Check sheet for the modelled part. Datum: model origin and axes. Units: mm. A direction names the side the tool comes from. Round coordinates to 2 decimals unless told otherwise and drop trailing zeros. Order: outer loops, then holes, each group sorted by start corner. A loop starts at its lowest first (then second) coordinate and runs counter-clockwise, first axis right, second up.
Q1. Mould release check, pull along Z, two halves, no side actions. Record for faces 1 (the cylindrical face through (-15.2, -5.73, 58.03)), 2 (the flat face through (14.3, 0, 27)): +Z half, -Z half, draft (parallel to the pull), parting line (faces both ways), or undercut.
Q2. Set-up check for faces 3 (the flat face through (-15.8, 0, -3)), 4 (the flat face through (0, 6.3, -3)), 5 (the cylindrical face through (-13.73, 4.7, 27.88)), 6 (the flat face through (0, 3.8, 28)): record each of +Z, -Z, +X, -X, +Y, -Y from which the full face is reachable in a straight line by a thin tool's end or side.
Q3. Cross-section at A-A on x = -6.5. Record the cut outline in (y, z), then the cut area to 3 significant figures.
Q4. Cross-section at D-D on y = 8. Record the cut outline in (x, z).
Q5. Cross-section at B-B on z = 35. Record the cut outline in (x, y).
Q6. Scan lines: probe 1 along X at (y, z) = (2, 53.5); probe 2 along Y at (x, z) = (-3, 37.5); probe 3 along Z at (x, y) = (-9, 5.75). Record each from-to range of solid material in increasing order.
Q7. Cross-section at C-C on y = -1. Record the cut outline in (x, z).
Q8. Depth check by flat-ended pin: P1, Ø8, axis at y = -0.5, z = 36.5, coming from the -X side; P2, Ø2, axis at x = 4, z = 58.5, coming from the -Y side; P3, Ø3, axis at y = 1, z = -3.5, coming from the +X side; P4, Ø6, axis at x = -1, y = 0, coming from the +Z side. Enter the tip coordinate at first touch or a pass-through.
from build123d import *

# Parameters (mm, degrees)
SKETCH1_W           = 28.6
SKETCH1_H           = 10.6
SKETCH1_W_2         = 25.6
SKETCH1_H_2         = 7.6
BOSS_EXTRUDE1_DEPTH = 55
SKETCH2_W           = 36.6
SKETCH2_H           = 18.6
SKETCH2_W_2         = 25.6
SKETCH2_H_2         = 7.6
BOSS_EXTRUDE3_DEPTH = 1
SKETCH3_W           = 31.6
SKETCH3_H           = 12.6
SKETCH3_W_2         = 25.6
SKETCH3_H_2         = 7.6
BOSS_EXTRUDE4_DEPTH = 4
FILLET1_R           = 2
FILLET2_R           = 2


with BuildPart() as part:
    # Sketch1 → Boss-Extrude1 (new body)
    with BuildSketch(Plane.XY):
        Rectangle(SKETCH1_W, SKETCH1_H)
        Rectangle(SKETCH1_W_2, SKETCH1_H_2, mode=Mode.SUBTRACT)
    extrude(amount=BOSS_EXTRUDE1_DEPTH)

    # Sketch2 → Boss-Extrude3 (add)
    with BuildSketch(Plane.XY.offset(55)):
        Rectangle(SKETCH2_W, SKETCH2_H)
        Rectangle(SKETCH2_W_2, SKETCH2_H_2, mode=Mode.SUBTRACT)
    boss_extrude3 = extrude(amount=BOSS_EXTRUDE3_DEPTH)

    # Sketch3 → Boss-Extrude4 (add)
    with BuildSketch(Plane.XY.offset(56)):
        Rectangle(SKETCH3_W, SKETCH3_H)
        Rectangle(SKETCH3_W_2, SKETCH3_H_2, mode=Mode.SUBTRACT)
    boss_extrude4 = extrude(amount=BOSS_EXTRUDE4_DEPTH)

    # Mirror1: Boss-Extrude3, Boss-Extrude4 across plane
    add(boss_extrude3.mirror(Plane(origin=(0, 0, 27.5), x_dir=(1, 0, 0), z_dir=(0, 0, -1))))
    add(boss_extrude4.mirror(Plane(origin=(0, 0, 27.5), x_dir=(1, 0, 0), z_dir=(0, 0, -1))))

    # Fillet1
    fillet1_edges = [part.edges().sort_by_distance(p)[0] for p in [
        (12.8, -3.8, 27.5),
        (12.8, 3.8, 27.5),
        (-12.8, 3.8, 27.5),
        (-12.8, -3.8, 27.5),
        (15.8, -6.3, 58),
        (15.8, 6.3, 58),
        (-15.8, 6.3, 58),
        (-15.8, -6.3, 58),
        (14.3, -5.3, 27.5),
        (-14.3, -5.3, 27.5),
        (-14.3, 5.3, 27.5),
        (14.3, 5.3, 27.5),
        (15.8, 6.3, -3),
        (15.8, -6.3, -3),
        (-15.8, -6.3, -3),
        (-15.8, 6.3, -3),
    ]]
    fillet(fillet1_edges, radius=FILLET1_R)

    # Fillet2
    fillet2_edges = [part.edges().sort_by_distance(p)[0] for p in [
        (18.3, -9.3, 55.5),
        (18.3, 9.3, 55.5),
        (-18.3, 9.3, 55.5),
        (-18.3, -9.3, 55.5),
        (18.3, 9.3, -0.5),
        (18.3, -9.3, -0.5),
        (-18.3, -9.3, -0.5),
        (-18.3, 9.3, -0.5),
    ]]
    fillet(fillet2_edges, radius=FILLET2_R)


solid = part.part
Results found:
1. face 1: draft
1. face 2: undercut
2. face 3: -Z, -X, +Y, -Y
2. face 4: -Z, +X, -X, +Y
2. face 5: -X, +Y
2. face 6: +Z, -Z
3. outline: (-9.3, -1) - (-6.3, -1) - (-6.3, -5) - (-3.8, -5) - (-3.8, 60) - (-6.3, 60) - (-6.3, 56) - (-9.3, 56) - (-9.3, 55) - (-5.3, 55) - (-5.3, 0) - (-9.3, 0) - close; (3.8, -5) - (6.3, -5) - (6.3, -1) - (9.3, -1) - (9.3, 0) - (5.3, 0) - (5.3, 55) - (9.3, 55) - (9.3, 56) - (6.3, 56) - (6.3, 60) - (3.8, 60) - close
3. area: 227 mm2
4. outline: (-18.17, -1) - (18.17, -1) - (18.17, 0) - (-18.17, 0) - close; (-18.17, 55) - (18.17, 55) - (18.17, 56) - (-18.17, 56) - close
5. outline: (-14.3, -3.3) arc R2 ccw to (-12.3, -5.3) - (12.3, -5.3) arc R2 ccw to (14.3, -3.3) - (14.3, 3.3) arc R2 ccw to (12.3, 5.3) - (-12.3, 5.3) arc R2 ccw to (-14.3, 3.3) - close; hole (-12.8, -1.8) arc R2 ccw to (-10.8, -3.8) - (10.8, -3.8) arc R2 ccw to (12.8, -1.8) - (12.8, 1.8) arc R2 ccw to (10.8, 3.8) - (-10.8, 3.8) arc R2 ccw to (-12.8, 1.8) - close
6. probe 1: x = -14.3 to -12.79, 12.79 to 14.3
6. probe 2: y = -5.3 to -3.8, 3.8 to 5.3
6. probe 3: z = -5 to 0, 55 to 60
7. outline: (-18.3, -1) - (-15.8, -1) - (-15.8, -5) - (-12.8, -5) - (-12.8, 60) - (-15.8, 60) - (-15.8, 56) - (-18.3, 56) - (-18.3, 55) - (-14.3, 55) - (-14.3, 0) - (-18.3, 0) - close; (12.8, -5) - (15.8, -5) - (15.8, -1) - (18.3, -1) - (18.3, 0) - (14.3, 0) - (14.3, 55) - (18.3, 55) - (18.3, 56) - (15.8, 56) - (15.8, 60) - (12.8, 60) - close
8. P1: stops at x = -14.3
8. P2: stops at y = -6.3
8. P3: stops at x = 15.8
8. P4: passes through
